```python
from build123d import *

# Parameters (mm, degrees)
SHELL_WALLS_DEPTH             = 68.58
SHELL_TOP_DEPTH               = 1.42
REAR_COOLING_FAN_CUTOUT_REACH = 146.493
REAR_COOLING_FAN_SKETCH_W     = 5
REAR_COOLING_FAN_SKETCH_H     = 92.06


with BuildPart() as part:
    # Shell → Shell Walls (new body)
    with BuildSketch(Plane.XY):
        with BuildLine():
            Line((-47.53, 56.53), (47.53, 56.53))
            ThreePointArc((47.53, 56.53), (53.893961031, 53.893961031), (56.53, 47.53))
            Line((56.53, 47.53), (56.53, -47.53))
            ThreePointArc((56.53, -47.53), (53.893961031, -53.893961031), (47.53, -56.53))
            Line((47.53, -56.53), (-47.53, -56.53))
            ThreePointArc((-47.53, -56.53), (-53.893961031, -53.893961031), (-56.53, -47.53))
            Line((-56.53, -47.53), (-56.53, 47.53))
            ThreePointArc((-56.53, 47.53), (-53.893961031, 53.893961031), (-47.53, 56.53))
        make_face()
        with BuildLine():
            Line((-47.53, 52.53), (47.53, 52.53))
            ThreePointArc((47.53, 52.53), (51.065533906, 51.065533906), (52.53, 47.53))
            Line((52.53, 47.53), (52.53, -47.53))
            ThreePointArc((52.53, -47.53), (51.065533906, -51.065533906), (47.53, -52.53))
            Line((47.53, -52.53), (-47.53, -52.53))
            ThreePointArc((-47.53, -52.53), (-51.065533906, -51.065533906), (-52.53, -47.53))
            Line((-52.53, -47.53), (-52.53, 47.53))
            ThreePointArc((-52.53, 47.53), (-51.065533906, 51.065533906), (-47.53, 52.53))
        make_face(mode=Mode.SUBTRACT)
    extrude(amount=SHELL_WALLS_DEPTH)

    # Sketch3 → Shell Top (add)
    with BuildSketch(Plane.XY.offset(68.58)):
        with BuildLine():
            Line((-56.53, 47.53), (-56.53, -47.53))
            ThreePointArc((-56.53, -47.53), (-53.893961031, -53.893961031), (-47.53, -56.53))
            Line((-47.53, -56.53), (47.53, -56.53))
            ThreePointArc((47.53, -56.53), (53.893961031, -53.893961031), (56.53, -47.53))
            Line((56.53, -47.53), (56.53, 47.53))
            ThreePointArc((56.53, 47.53), (53.893961031, 53.893961031), (47.53, 56.53))
            Line((47.53, 56.53), (-47.53, 56.53))
            ThreePointArc((-47.53, 56.53), (-53.893961031, 53.893961031), (-56.53, 47.53))
        make_face()
    extrude(amount=SHELL_TOP_DEPTH)

    # Rear-Cooling Fan Sketch → Rear-Cooling Fan Cutout (cut, up to next)
    with BuildSketch(Plane.ZY.offset(56.53), mode=Mode.PRIVATE) as rear_cooling_fan_cutout_sk1:
        with Locations((65.5, 0)):
            Rectangle(REAR_COOLING_FAN_SKETCH_W, REAR_COOLING_FAN_SKETCH_H)
    rear_cooling_fan_cutout_tool1 = extrude(rear_cooling_fan_cutout_sk1.sketch, amount=-REAR_COOLING_FAN_CUTOUT_REACH, mode=Mode.PRIVATE) & part.part
    add(rear_cooling_fan_cutout_tool1.solids().sort_by_distance((-56.53, 0, 65.5))[0], mode=Mode.SUBTRACT)


solid = part.part
```
Source: CAD feature listing. Evaluate the final solid. Frame: model axes, mm. A direction names the side the tool comes from. Coordinates: 2 decimals unless noted, no trailing zeros. Order: outer loops, then holes, each group sorted by start corner. A loop starts at its lowest first (then second) coordinate and runs counter-clockwise, first axis right, second up. Notation, with made-up numbers: M -2,65 L 3,65 A20 ccw 3,99 Z; hole C -40,66.25 d8. An arc over 180 degrees is marked long. Write each question's results on one line, items separated by ' | '. Start each with the question number.
1) Contact query for flat-ended pins moving along their axis: pin 1 Ø3 at (x, z) = (-54.5, 66.5) entering from -Y; pin 2 Ø1 at (x, y) = (-9.5, -16.5) entering from -Z; pin 3 Ø3 at (x, z) = (-54, 66.5) entering from +Y; pin 4 Ø4.5 at (x, y) = (-55, 11) entering from -Z. Output: stop coordinate, or through.
2) Section query C-C (x = 46). Return the cut outline in (y, z).
3) Access query for faces 4 (the face through (52.53, 1, 34)), 5 (the face through (1, 56.53, 35)), 6 (the face through (-55, 46.03, 65)). Directions: +Z, -Z, +X, -X, +Y, -Y. A direction counts if a zero-diameter tool reaches every point of the face in a straight line with its end or side. Return the directions, or none.
4) Section query A-A (y = -9.5). Return the cut outline in (x, z), plus the area to 3 significant figures.
5) Section query B-B (z = 8). Return the cut outline in (x, y).
6) Draft query along Z for faces 1 (the face through (-1, 1, 68.58)), 2 (the face through (-55, -1, 63)), 3 (the face through (-52.53, -1, 34)). Return one class per face: released by +Z, released by -Z, zero draft, split by the parting line, or undercut.
7) Section query D-D (y = 49.5). Return the cut outline in (x, z).
8) Line query: line 1 (X direction, y = 8, z = 17); line 2 (X direction, y = 44.5, z = 64.5). Output: solid intervals per line, ascending. Write a range as from..to.
Answers:
1) pin 1: stops at y = -54.68 | pin 2: stops at z = 68.58 | pin 3: stops at y = 55.03 | pin 4: stops at z = 0
2) outline: M -56.53,0 L -52.53,0 L -52.53,68.58 L 52.53,68.58 L 52.53,0 L 56.53,0 L 56.53,70 L -56.53,70 Z
3) face 4: -Z | face 5: +Z, -Z, +X, -X, +Y | face 6: -X
4) outline: M -56.53,0 L -52.53,0 L -52.53,63 L -56.53,63 Z; M -56.53,68 L -52.53,68 L -52.53,68.58 L 52.53,68.58 L 52.53,0 L 56.53,0 L 56.53,70 L -56.53,70 Z | area: 689 mm^2
5) outline: M -56.53,-47.53 A9 ccw -47.53,-56.53 L 47.53,-56.53 A9 ccw 56.53,-47.53 L 56.53,47.53 A9 ccw 47.53,56.53 L -47.53,56.53 A9 ccw -56.53,47.53 Z; hole M -52.53,-47.53 A5 ccw -47.53,-52.53 L 47.53,-52.53 A5 ccw 52.53,-47.53 L 52.53,47.53 A5 ccw 47.53,52.53 L -47.53,52.53 A5 ccw -52.53,47.53 Z
6) face 1: released by -Z | face 2: undercut | face 3: zero draft
7) outline: M -56.31,0 L -52.13,0 L -52.13,68.58 L 52.13,68.58 L 52.13,0 L 56.31,0 L 56.31,70 L -56.31,70 Z
8) line 1: x = -56.53..-52.53, 52.53..56.53 | line 2: x = 52.53..56.53
